CAD build for the part. Positions are in the model's coordinates, mm. A direction names the side the tool comes from. Round coordinates to 2 decimals unless told otherwise and drop trailing zeros. Loops run counter-clockwise (first coordinate to the right, second up) from the corner with the lowest first, then second, coordinate; pieces in that order, holes last.
from build123d import *

# Parameters (mm, degrees)
ESQUISSE1_W             = 350
ESQUISSE1_H             = 350
BOSS_EXTRU_1_DEPTH      = 26
ESQUISSE2_W             = 340
ESQUISSE2_H             = 340
ESQUISSE2_W_2           = 295
ESQUISSE2_H_2           = 295
ENL_V_MAT_EXTRU_1_DEPTH = 20
ESQUISSE3_W             = 295
ESQUISSE3_H             = 295
ENL_V_MAT_EXTRU_2_DEPTH = 249.849352018
ESQUISSE4_W             = 50
ESQUISSE4_H             = 12
ESQUISSE4_W_2           = 12
ESQUISSE4_H_2           = 50
BOSS_EXTRU_2_DEPTH      = 5


with BuildPart() as part:
    # Esquisse1 → Boss.-Extru.1 (new body)
    with BuildSketch(Plane.XY):
        Rectangle(ESQUISSE1_W, ESQUISSE1_H)
    extrude(amount=BOSS_EXTRU_1_DEPTH)

    # Esquisse2 → Enlèv. mat.-Extru.1 (cut)
    with BuildSketch(Plane.XY.offset(26)):
        Rectangle(ESQUISSE2_W, ESQUISSE2_H)
        Rectangle(ESQUISSE2_W_2, ESQUISSE2_H_2, mode=Mode.SUBTRACT)
    extrude(amount=-ENL_V_MAT_EXTRU_1_DEPTH, mode=Mode.SUBTRACT)

    # Esquisse3 → Enlèv. mat.-Extru.2 (cut, through all)
    with BuildSketch(Plane.XY.offset(26)):
        Rectangle(ESQUISSE3_W, ESQUISSE3_H)
    extrude(amount=-ENL_V_MAT_EXTRU_2_DEPTH, mode=Mode.SUBTRACT)

    # Esquisse4 → Boss.-Extru.2 (add)
    with BuildSketch(Plane.XY):
        with Locations((-200, 0)):
            Rectangle(ESQUISSE4_W, ESQUISSE4_H)
        with Locations((200, 0)):
            Rectangle(ESQUISSE4_W, ESQUISSE4_H)
        with Locations((0, 200)):
            Rectangle(ESQUISSE4_W_2, ESQUISSE4_H_2)
        with Locations((0, -200)):
            Rectangle(ESQUISSE4_W_2, ESQUISSE4_H_2)
    extrude(amount=BOSS_EXTRU_2_DEPTH)


solid = part.part
Item 1: Cut at A-A (z = 14). List the corners of the cut face in (x, y).
Verdict:
outline: (-175, -175) - (175, -175) - (175, 175) - (-175, 175) - close; hole (-170, -170) - (170, -170) - (170, 170) - (-170, 170) - close
Item 2: Wall check: L1, parallel to X at y = 103.5, z = 13; L2, parallel to X at y = -207, z = 2. Give the ranges that are in metal, low to high.
Verdict:
L1: x = -175 to -170, 170 to 175
L2: x = -6 to 6
Item 3: 3-axis set-ups, long thin cutter, end or side, ignore diameter. For faces 1 (the flat face through (200, 0, 5)), 2 (the flat face through (-200, 0, 5)), 3 (the flat face through (-2, -170, 16)), 4 (the flat face through (0, 200, 5)): which of +Z, -Z, +X, -X, +Y, -Y reach the whole face in a straight line?
Verdict:
face 1: +Z, +X, +Y, -Y
face 2: +Z, -X, +Y, -Y
face 3: +Z
face 4: +Z, +X, -X, +Y
Item 4: Mould opens along X. For faces 5 (the flat face through (149, 2, 6)), 6 (the flat face through (-2, -175, 13)) say: released by +X, released by -X, zero draft, split by the parting line, or undercut.
Verdict:
face 5: undercut
face 6: zero draft
Item 5: Flat gauge pins, fed straight in: P1, Ø5.5, axis at x = -192.5, z = 3, coming from the +Y side; P2, Ø2.5, axis at y = 200.5, z = 3.5, coming from the -X side; P3, Ø12, axis at x = -4, z = 15, coming from the -Y side. Where does each tip first touch, or does it go through?
Verdict:
P1: stops at y = 6
P2: stops at x = -6
P3: stops at y = -175
Item 6: Cut at D-D (y = 161.5). List the corners of the cut face in (x, z), plus the area to 3 significant figures.
Verdict:
outline: (-175, 0) - (175, 0) - (175, 26) - (170, 26) - (170, 6) - (-170, 6) - (-170, 26) - (-175, 26) - close
area: 2,300 mm2
Item 7: Cut at B-B (x = -57). List the corners of the cut face in (y, z), plus the area to 3 significant figures.
Verdict:
outline: (-175, 0) - (-147.5, 0) - (-147.5, 6) - (-170, 6) - (-170, 26) - (-175, 26) - close; (147.5, 0) - (175, 0) - (175, 26) - (170, 26) - (170, 6) - (147.5, 6) - close
area: 530 mm2
